Can you work these out from the drawing? Everything is in mm from the part's minimum corner. Coordinates: 2 decimals unless noted, no trailing zeros. Order: outer loops, then holes, each group sorted by start corner. A loop starts at its lowest first (then second) coordinate and runs counter-clockwise, first axis right, second up. Notation, with made-up numbers: (61.5, 0) -> (89.5, 0) arc R17 cw to (89.5, 10) -> close; hole circle Ø1 at (10, 79.5). An arc over 180 degrees is marked (long way). Use a Markdown table: item, result. Add a question column.
1) Will these pins go through, and if not, where does the flat tip stop? pin 1 Ø1.5 at (x, y) = (86, 36.5) entering from +Z; pin 2 Ø4 at (y, z) = (19.5, 27) entering from -X; pin 3 Ø1 at (x, z) = (42, 11) entering from +Y; pin 4 Ø1.5 at (x, z) = (52, 32) entering from +Y.
2) If we section it at A-A (y = 19.5): Write out the boundary of the cut face in (x, z), plus the area to 3 significant figures.
3) If we section it at C-C (x = 71.5): Write out the boundary of the cut face in (y, z).
4) If we section it at D-D (y = 45): Write out the boundary of the cut face in (x, z).
5) If we section it at B-B (z = 31): Write out the boundary of the cut face in (x, y), plus the area to 3 significant figures.
6) Thinking about a two-plate mould opening in Z: for the marked faces 1, 2, 3 and 4, which applies, +Z half, -Z half, draft (parallel to the pull), parting line (faces both ways), or undercut?
7) If I drill on L1, parallel to Z at x = 62, y = 22; L2, parallel to Z at x = 22, y = 37.5; L3, parallel to Y at x = 58, z = 13, over which ranges is the centre line in solid material (lowest first)? Write a range as [from, to].
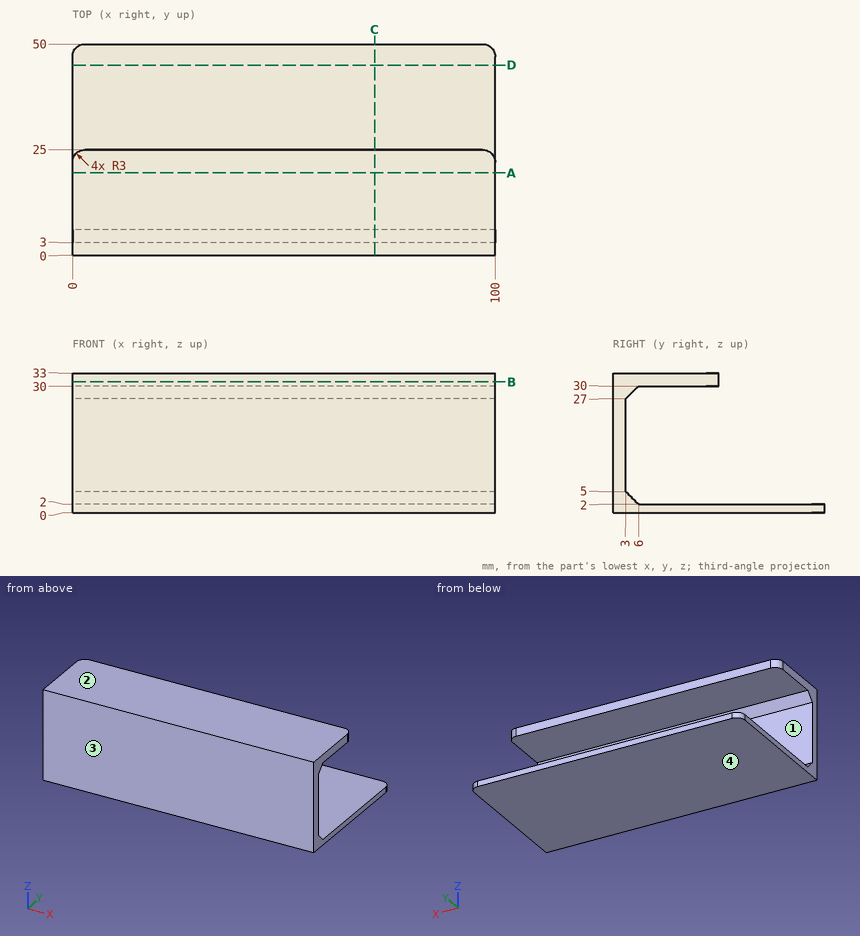
Answer sheet:
| question | item | result |
|---|---|---|
| 1 | pin 1 | z = 2 |
| 1 | pin 2 | through |
| 1 | pin 3 | y = 3 |
| 1 | pin 4 | y = 25 |
| 2 | outline | (0, 0) -> (100, 0) -> (100, 2) -> (0, 2) -> close; (0, 30) -> (100, 30) -> (100, 33) -> (0, 33) -> close |
| 2 | area | 500 mm2 |
| 3 | outline | (0, 0) -> (50, 0) -> (50, 2) -> (6, 2) -> (3, 5) -> (3, 27) -> (6, 30) -> (25, 30) -> (25, 33) -> (0, 33) -> close |
| 4 | outline | (0, 0) -> (100, 0) -> (100, 2) -> (0, 2) -> close |
| 5 | outline | (0, 0) -> (100, 0) -> (100, 22) arc R3 ccw to (97, 25) -> (3, 25) arc R3 ccw to (0, 22) -> close |
| 5 | area | 2,500 mm2 |
| 6 | face 1 | undercut |
| 6 | face 2 | +Z half |
| 6 | face 3 | draft |
| 6 | face 4 | -Z half |
| 7 | L1 | [0, 2], [30, 33] |
| 7 | L2 | [0, 2] |
| 7 | L3 | [0, 3] |
